Model file for the job. Use its own axes, mm. Face numbers are marked on the shaded views. A direction names the side the tool comes from. Give positions to 0.01 mm unless a question says otherwise; leave off trailing zeros. Order: outer loops, then holes, each group sorted by start corner. A loop starts at its lowest first (then second) coordinate and runs counter-clockwise, first axis right, second up. Notation, with made-up numbers: (32, 85.5) - (74, 85.5) arc R26 cw to (74, 108.5) - close; hole circle Ø1 at (83, -1). An arc over 180 degrees is marked (long way). Use CSV: the item, a comma, the result in double quotes. Start each with the question number.
(1) Drop flat-ended pins along their axis: pin 1 Ø2 at (y, z) = (-4, -2) entering from +X; pin 2 Ø2 at (x, z) = (31, -4.5) entering from +Y; pin 3 Ø1.6 at (y, z) = (-1.5, -3) entering from -X; pin 4 Ø6 at (x, y) = (31.5, 2) entering from -Z. Give the stop position or say it passes through.
(2) Probe L1, parallel to Z at x = 5.4, y = 0; L2, parallel to X at y = -2.75, z = -5; L3, parallel to Z at x = 6.6, y = 0. List the from-to ranges inside material, lowest first.
(3) Band-saw the part on A-A, the plane x = 18.5. Give the cut face in (y, z).
(4) Tool access for the marked faces 4, 5 and 6: list every direction of +Z, -Z, +X, -X, +Y, -Y with a clear straight run to the whole face (end or side of a thin tool).
(5) Pull direction Z, two halves, no side cores. Call the marked faces 1, 2 and 3: +Z half, -Z half, draft (parallel to the pull), parting line (faces both ways), or undercut.
from build123d import *

# Parameters (mm, degrees)
FILLET1_R   = 0.4
FILLET2_R   = 1
HEX_2_DEPTH = 3.65


with BuildPart() as part:
    # BodySke → Base-Revolve (revolve)
    with BuildSketch(Plane.XY):
        Polygon((0, 0), (0, 8), (6.5, 8), (6.5, 5), (35.672, 5), (36.5, 4.172), (36.5, 0), align=None)
    revolve(axis=Axis((-31.75, 0, 0), (1, 0, 0)))

    # Fillet1
    fillet1_edges = [part.edges().sort_by_distance(p)[0] for p in [
        (6.5, -5, 0),
    ]]
    fillet(fillet1_edges, radius=FILLET1_R)

    # Fillet2
    fillet2_edges = [part.edges().sort_by_distance(p)[0] for p in [
        (0, -8, 0),
    ]]
    fillet(fillet2_edges, radius=FILLET2_R)

    # HexSke → Hex 2 (cut)
    with BuildSketch(Plane(origin=(0, 0, 0), x_dir=(0, 0.5, 0.866025404), z_dir=(-1, 0, 0))):
        Polygon((2.359919225, 4.0875), (-2.359919225, 4.0875), (-4.719838451, 0), (-2.359919225, -4.0875), (2.359919225, -4.0875), (4.719838451, 0), align=None)
    extrude(amount=-HEX_2_DEPTH, mode=Mode.SUBTRACT)

    # PilotSke → Hex-PreBroach (revolve, cut)
    with BuildSketch(Plane.XY):
        Polygon((0, 4.0875), (3.65, 4.0875), (4.544892917, 2.5375), (7.86, 2.5375), (9.325026308, 0), (0, 0), align=None)
    revolve(axis=Axis((0, 0, 0), (1, 0, 0)), mode=Mode.SUBTRACT)


solid = part.part
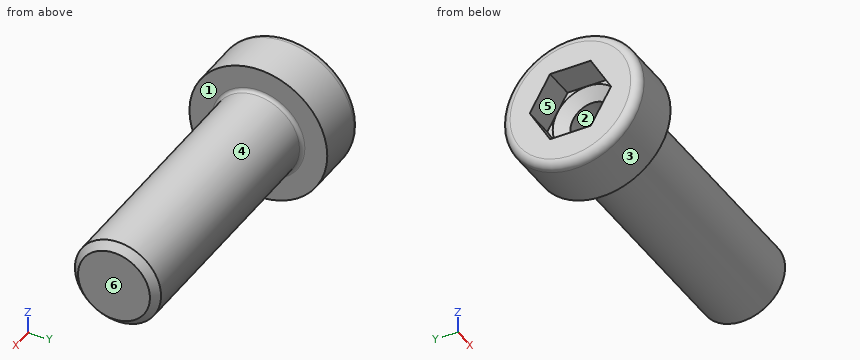
Answer block:
1,pin 1,"stops at x = 36.5"
1,pin 2,"stops at y = 3.57"
1,pin 3,"stops at x = 3.65"
1,pin 4,"stops at z = -5"
2,L1,"z = -8 to -2.54, 2.54 to 8"
2,L2,"x = 0 to 6.5"
2,L3,"z = -5.14 to -2.54, 2.54 to 5.14"
3,outline,"circle Ø10 at (0, 0)"
4,face 4,"+X"
4,face 5,"-X"
4,face 6,"+Z, -Z, +X, +Y, -Y"
5,face 1,"draft"
5,face 2,"undercut"
5,face 3,"parting line"
